Model file for the job. Use its own axes, mm. A direction names the side the tool comes from. Round coordinates to 2 decimals unless told otherwise and drop trailing zeros. Put each result on its own line as item: value. Start each with the question number.
Q1. Pull direction X, two halves, no side cores. Call faces 6 (the face through (20.645, 0.764, -0.724)), 7 (the face through (99.278, 0.764, -89.446)), 8 (the face through (10.414, 2, 1)): released by +X, released by -X, zero draft, split by the parting line, or undercut.
Q2. Flat gauge pins, fed straight in: P1, Ø2, axis at x = 88, y = 2, coming from the +Z side; P2, Ø4, axis at x = 17.5, y = 5.5, coming from the -Z side; P3, Ø3, axis at x = 43.5, y = 6, coming from the +Z side; P4, Ø1, axis at y = 1.5, z = -67, coming from the -X side. Where does each tip first touch, or does it go through?
Q3. 3-axis set-ups, long thin cutter, end or side, ignore diameter. For faces 1 (the face through (49.458, 1.878, -55.114)), 2 (the face through (15.494, 2, 1)), 3 (the face through (106, 2, -87.63)), 4 (the face through (40, 2, -87.63)), 5 (the face through (56, 2, 0)): which of +Z, -Z, +X, -X, +Y, -Y reach the whole face in a straight line?
Q4. Probe L1, parallel to X at y = 1.75, z = -72; L2, parallel to Y at x = 42, z = -77; L3, parallel to Z at x = 73.5, y = 2.5. List the from-to ranges inside material, lowest first.
Autodesk Inventor part; units mm, degrees
ref_plane "Work Plane1" through (49.784, 0, -43.815) normal (0, 0, -1) x (-1, 0, 0)
ref_plane "YZ Plane" through (0, 0, 0) normal (1, 0, 0) x (0, 1, 0)
ref_plane "XZ Plane" through (0, 0, 0) normal (0, 1, 0) x (-1, 0, 0)
sketch "Sketch1" plane through (0, 0, 0) normal (0, 1, 0) x (-1, 0, 0)
  line L0 (0, 0) -> (-112.268, 0)
  line L1 (-112.268, 0) -> (-112.268, -87.63)
  line L2 (-112.268, -87.63) -> (0, -87.63)
  line L3 (0, -87.63) -> (0, 0)
  dimension "d0" = 87.63
  dimension "d1" = 112.268
extrude "Extrusion1" add sketch "Sketch1" along normal blind 3.81
sketch "Sketch2" plane through (0, 3.81, 0) normal (0, 1, 0) x (1, 0, 0)
  line L0 (4.318, 83.312) -> (107.95, 83.312)
  line L1 (107.95, 83.312) -> (107.95, 4.318)
  line L2 (107.95, 4.318) -> (4.318, 4.318)
  line L3 (4.318, 4.318) -> (4.318, 83.312)
  line L4 (112.268, 87.63) -> (0, 87.63)
  line L5 (0, 87.63) -> (0, 0)
  line L6 (0, 0) -> (112.268, 0)
  line L7 (112.268, 0) -> (112.268, 87.63)
  line L8 (8.128, 79.502) -> (104.14, 79.502)
  line L9 (104.14, 79.502) -> (104.14, 8.128)
  line L10 (104.14, 8.128) -> (8.128, 8.128)
  line L11 (8.128, 8.128) -> (8.128, 79.502)
  dimension "d4" = 4.318
  dimension "d5" = 4.318
  dimension "d6" = 4.318
  dimension "d7" = 4.318
  dimension "d8" = 3.81
extrude "Extrusion2" add sketch "Sketch2" along normal blind 3.81 contours L0 L1 L2 L3
chamfer "Chamfer1" distance 3.81 angle 45 4 edges at (8.128, 7.62, -43.815) (56.134, 7.62, -79.502) (104.14, 7.62, -43.815) (56.134, 7.62, -8.128)
sketch "Sketch3" plane through (0, 0, 0) normal (0, -1, 0) x (1, 0, 0)
  arc A0 (63.754, -53.975) -> (48.514, -53.975) centre (56.134, -43.815) ccw
  line L0 (112.268, 0) -> (112.268, -87.63)
  line L1 (112.268, -87.63) -> (0, -87.63)
  line L2 (49.784, -56.515) -> (49.784, -87.63)
  line L3 (62.484, -56.515) -> (62.484, -87.63)
  arc A1 (49.784, -56.515) -> (48.514, -53.975) centre (46.609, -56.515) ccw
  arc A2 (63.754, -53.975) -> (62.484, -56.515) centre (65.659, -56.515) ccw
  point P0 (0, 0)
  point P1 (112.268, -43.815)
  point P2 (56.134, -87.63)
  point P3 (43.434, -43.815)
  point P4 (43.434, -87.63)
  point P5 (68.834, -43.815)
  point P6 (68.834, -87.63)
  point P7 (49.784, -54.8135)
  point P8 (62.484, -54.8135)
  point P9 (56.134, -87.63)
  dimension "d14" = 25.4
  dimension "d17" = 12.7
  dimension "d18" = 6.35
  dimension "d19" = 3.175
extrude "Extrusion3" cut sketch "Sketch3" against normal blind 62.865
fillet "Fillet1" radius 2.54 4 edges at (0, 1.905, -87.63) (112.268, 1.905, -87.63) (112.268, 1.905, 0) (0, 1.905, 0)
sketch "Sketch4" plane through (49.784, 0, -87.63) normal (0, 0, -1) x (-1, 0, 0)
  line L0 (0, 0) -> (47.244, 0)
  line L1 (45.466, 3.81) -> (0, 3.81)
  line L2 (39.37, 0) -> (34.29, 0)
  line L3 (34.29, 0) -> (34.29, 3.81)
  line L4 (34.29, 3.81) -> (39.37, 3.81)
  line L5 (39.37, 3.81) -> (39.37, 0)
  line L6 (24.13, 3.81) -> (19.05, 3.81)
  line L7 (19.05, 3.81) -> (19.05, 0)
  line L8 (19.05, 0) -> (24.13, 0)
  line L9 (24.13, 0) -> (24.13, 3.81)
  line L10 (-31.75, 3.81) -> (-36.83, 3.81)
  line L11 (-36.83, 3.81) -> (-36.83, 0)
  line L12 (-36.83, 0) -> (-31.75, 0)
  line L13 (-31.75, 0) -> (-31.75, 3.81)
  line L14 (-12.7, 3.81) -> (-58.166, 3.81)
  line L15 (-46.99, 3.81) -> (-52.07, 3.81)
  line L16 (-52.07, 3.81) -> (-52.07, 0)
  line L17 (-52.07, 0) -> (-46.99, 0)
  line L18 (-46.99, 0) -> (-46.99, 3.81)
  line L19 (45.466, 7.62) -> (-58.166, 7.62)
  point P0 (49.784, 0)
  point P1 (34.29, 1.905)
  point P2 (39.37, 1.905)
  point P3 (19.05, 1.905)
  point P4 (24.13, 1.905)
  point P5 (-36.83, 1.905)
  point P6 (-31.75, 1.905)
  point P7 (-52.07, 1.905)
  point P8 (-46.99, 1.905)
  point P9 (-6.35, 7.62)
  point P10 (-52.07, 3.81)
  point P11 (19.05, 3.81)
  point P12 (19.05, 0)
  dimension "d21" = 5.08
  dimension "d22" = 5.08
  dimension "d23" = 5.08
  dimension "d24" = 5.08
  dimension "d25" = 10.16
  dimension "d26" = 10.16
  dimension "d27" = 50.8
  dimension "d28" = 25.4
extrude "Extrusion4" add sketch "Sketch4" along normal blind 2.54 contours L7 L1 L9 L0 | L3 L1 L5 L0 | L13 L12 L11 L10 | L18 L17 L16 L14
ref_plane "Work Plane1" through (49.784, 0, -43.815) normal (0, 0, -1) x (-1, 0, 0)
mirror "Mirror1" about plane through (49.784, 0, -43.815) normal (0, 0, -1) of "Extrusion4"
fillet "Fillet2" radius 2.54 12 edges at (12.954, 0, -90.17) (20.574, 0, -87.63) (28.194, 0, -90.17) (91.694, 0, -87.63) (99.314, 0, -90.17) (84.074, 0, 2.54) (91.694, 0, 0) (99.314, 0, 2.54) (12.954, 0, 2.54) (20.574, 0, 0) (28.194, 0, 2.54) (84.074, 0, -90.17)
equation "\"d5\" = d4"
equation "\"d6\" = d4"
equation "\"d7\" = d4"
properties part number "Janus wire holder lid"
Ans:
1. face 6: undercut
1. face 7: zero draft
1. face 8: released by -X
2. P1: stops at z = 0
2. P2: stops at z = -87.63
2. P3: stops at z = -4.32
2. P4: stops at x = 0
3. face 1: +Y, -Y
3. face 2: +Z, -Y
3. face 3: -Z, +X, +Y, -Y
3. face 4: -Z, +Y, -Y
3. face 5: +Z, +Y, -Y
4. L1: x = 0 to 49.78, 62.48 to 112.27
4. L2: y = 0 to 3.81
4. L3: z = -87.63 to 0
